Here's how the part is built. I have some questions about the finished solid (model axes, mm). Face numbers are marked on the shaded views. Give positions to 0.01 mm unless a question says otherwise; leave off trailing zeros. Loops run counter-clockwise (first coordinate to the right, second up) from the corner with the lowest first, then second, coordinate; pieces in that order, holes last.
Q1. I need wall thicknesses on probe 1 along Z at (x, y) = (-72, -58.5); probe 2 along Y at (x, z) = (0, 110); probe 3 along Y at (x, z) = (70, 2.3). Which ranges of each line are inside material? Lowest first, please.
Q2. I'm going to push flat-ended pins straight in: P1, Ø5, axis at x = 45, z = 85, coming from the +Y side; P2, Ø12, axis at x = 9, y = 73.5, coming from the +Z side; P3, Ø4, axis at x = -120, z = 137, coming from the -Y side. Where does each tip first touch, or does it pass through?
Q3. Suppose I cut it at D-D (z = 106). List the corners of the cut face in (x, y) for me, and give its area (3 significant figures).
Q4. Thinking about a two-plate mould opening in Y: for the marked faces 1, 2 and 3, which applies, pulls with the +Y half, pulls with the -Y half, needs draft (parallel to the pull), parting line crosses it, or undercut?
Q5. Suppose I cut it at C-C (x = 0). List the corners of the cut face in (y, z) for me, and give its area (3 significant figures).
Q6. Suppose I cut it at A-A (y = 70). List the corners of the cut face in (x, z) for me (3 decimals).
Q7. Suppose I cut it at B-B (x = 63.5). List the corners of the cut face in (y, z) for me.
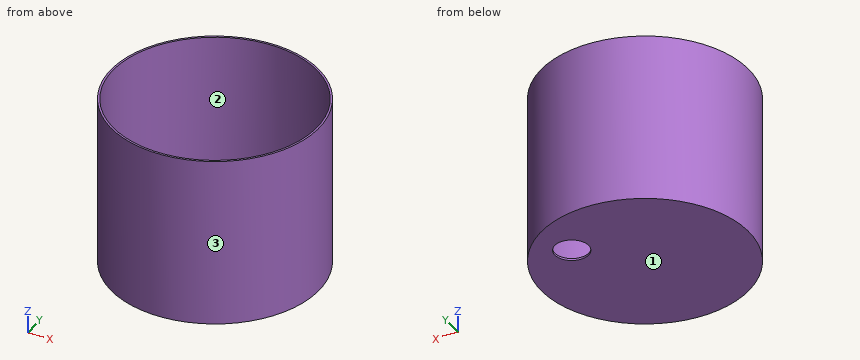
```python
from build123d import *

# Parameters (mm, degrees)
F0_R     = 153
F1_DEPTH = 250
F2_T     = -3
F3_R     = 25
F4_DEPTH = 25


with BuildPart() as f1:
    # F0 (on Top) → F1 (new body)
    with BuildSketch(Plane.XY):
        Circle(F0_R)
    extrude(amount=F1_DEPTH)

    # F2
    f2_openings = [f1.faces().sort_by_distance(p)[0] for p in [
        (0, 0, 250),
    ]]
    offset(amount=F2_T, openings=f2_openings)

    # F3 (on face) → F4 (cut)
    with BuildSketch(Plane.XY.offset(3)):
        with Locations((70, 70)):
            Circle(F3_R)
    extrude(amount=-F4_DEPTH, mode=Mode.SUBTRACT)


solid = f1.part
```
Solutions:
1. probe 1: z = 0 to 3
1. probe 2: y = -153 to -150, 150 to 153
1. probe 3: y = -136.05 to 45, 95 to 136.05
2. P1: stops at y = 146.98
2. P2: stops at z = 3
2. P3: stops at y = -97.39
3. outline: circle Ø306 at (0, 0); hole circle Ø300 at (0, 0)
3. area: 2,860 mm2
4. face 1: needs draft
4. face 2: undercut
4. face 3: parting line crosses it
5. outline: (-153, 0) - (153, 0) - (153, 250) - (150, 250) - (150, 3) - (-150, 3) - (-150, 250) - (-153, 250) - close
5. area: 2,400 mm2
6. outline: (-136.048, 0) - (45, 0) - (45, 3) - (-132.665, 3) - (-132.665, 250) - (-136.048, 250) - close; (95, 0) - (136.048, 0) - (136.048, 250) - (132.665, 250) - (132.665, 3) - (95, 3) - close
7. outline: (-139.2, 0) - (45.86, 0) - (45.86, 3) - (-135.9, 3) - (-135.9, 250) - (-139.2, 250) - close; (94.14, 0) - (139.2, 0) - (139.2, 250) - (135.9, 250) - (135.9, 3) - (94.14, 3) - close
